from build123d import *

# Parameters (mm, degrees)
F1_DEPTH = 10.16
F2_R     = 1.892747
F3_DEPTH = 14.986
F5_D     = 6.35


with BuildPart() as f1:
    # F0 (on Top) → F1 (new body)
    with BuildSketch(Plane.XY):
        Polygon((7.914659, 62.022142), (-7.914659, 62.022142), (-7.626853, -11.943939), (-12.51955, -47.344048), (-7.626853, -75.836815), (7.914659, -75.836815), (12.231744, -47.631852), (7.914659, -11.943939), align=None)
    extrude(amount=F1_DEPTH)

    # F2 (on face) → F3 (join)
    with BuildSketch(Plane(origin=(0, 62.022142, 0), x_dir=(-1, 0, 0), z_dir=(0, 1, 0))):
        with Locations((0, 5.900018)):
            Circle(F2_R)
    extrude(amount=F3_DEPTH)

    # F5 (through all)
    with Locations(Plane.XY.offset(10.16)):
        with Locations((0, -34.430573)):
            Hole(F5_D / 2)


solid = f1.part
The model under review builds one solid part; all positions refer to its coordinate system, in mm. A direction names the side the tool comes from. Round coordinates to 2 decimals unless told otherwise and drop trailing zeros. Order: outer loops, then holes, each group sorted by start corner. A loop starts at its lowest first (then second) coordinate and runs counter-clockwise, first axis right, second up. Notation, with made-up numbers: (10.25, -19) -> (41.25, -19) arc R13 cw to (41.25, -15) -> close; hole circle Ø5 at (16, 82.25). An arc over 180 degrees is marked (long way). Use CSV: the item, a comma, the result in double quotes. Start each with the question number.
(1) Wall thickness on probe 1 along Y at (x, z) = (0, 7.5); probe 2 along Y at (x, z) = (0, 3); probe 3 along X at (y, z) = (-34, 2.5): over which ranges is each line inside the solid? List them lowest first. Write a range as from..to.
(2) Consider section A-A on x = 0. Write out the cut boundary in (y, z).
(3) Mouldability with a two-part tool opening along X and no side actions: class faces 4 (the face through (-10.04, -29.4, 5.01)), 5 (the face through (2, 62.022, 5)), 6 (the face through (0.69, -37.53, 5.01)) as pulls with the +X half, pulls with the -X half, needs draft (parallel to the pull), parting line crosses it, or undercut.
(4) Insertion check: pin 1 (3 mm diameter, centred on y = 12, z = 4.5, fed in from +X); pin 2 (6 mm diameter, centred on y = -60.5, z = 3, fed in from -X); pin 3 (5 mm diameter, centred on x = 0, y = -34.43, fed in from +Z); pin 4 (1 mm diameter, centred on y = -52.5, z = 2, fed in from +X). Each pin has a flat end and moves straight along its axis. Give the tip position at first contact, or say it passes through.
(5) Tool access review of faces 1 (the face through (1.395, 69.41, 7.179)), 2 (the face through (7.915, 25, 5)), 3 (the face through (-10.107, -61.391, 5.009)): name each direction out of +Z, -Z, +X, -X, +Y, -Y from which nothing blocks a thin tool from reaching the whole face with its end or side.
(6) Consider section D-D on x = -5.5. Write out the cut boundary in (y, z).
(7) Consider section B-B on z = 2.25. Write out the cut boundary in (x, y) (3 decimals).
(8) Consider section C-C on y = -55. Write out the cut boundary in (x, z), and give its area (3 significant figures).
Responses:
1,probe 1,"-75.84..-37.61, -31.26..77.01"
1,probe 2,"-75.84..-37.61, -31.26..62.02"
1,probe 3,"-10.68..-3.15, 3.15..10.58"
2,outline,"(-75.84, 0) -> (-37.61, 0) -> (-37.61, 10.16) -> (-75.84, 10.16) -> close; (-31.26, 0) -> (62.02, 0) -> (62.02, 4.01) -> (77.01, 4.01) -> (77.01, 7.79) -> (62.02, 7.79) -> (62.02, 10.16) -> (-31.26, 10.16) -> close"
3,face 4,"pulls with the -X half"
3,face 5,"needs draft"
3,face 6,"undercut"
4,pin 1,"x = 7.91"
4,pin 2,"x = -10.78"
4,pin 3,"through"
4,pin 4,"x = 11.56"
5,face 1,"+Y"
5,face 2,"+Z, -Z, +X, +Y"
5,face 3,"+Z, -Z, -X, -Y"
6,outline,"(-75.84, 0) -> (62.02, 0) -> (62.02, 10.16) -> (-75.84, 10.16) -> close"
7,outline,"(-12.52, -47.344) -> (-7.627, -75.837) -> (7.915, -75.837) -> (12.232, -47.632) -> (7.915, -11.944) -> (7.915, 62.022) -> (-7.915, 62.022) -> (-7.627, -11.944) -> close; hole circle Ø6.35 at (0, -34.431)"
8,outline,"(-11.2, 0) -> (11.1, 0) -> (11.1, 10.16) -> (-11.2, 10.16) -> close"
8,area,"227 mm²"
